Source: CAD feature listing. Evaluate the final solid. Frame: model axes, mm. Face numbers are marked on the shaded views. A direction names the side the tool comes from. Give positions to 0.01 mm unless a question says otherwise; leave off trailing zeros. Loops run counter-clockwise (first coordinate to the right, second up) from the corner with the lowest first, then second, coordinate; pieces in that order, holes last. Notation, with made-up numbers: M 50,28.25 L 63,28.25 A17 ccw 63,50.25 Z; hole C 7,29.5 d8. An arc over 180 degrees is marked long. Put each result on its own line as item: value.
from build123d import *

# Parameters (mm, degrees)
F2_SIZE  = 1
F3_R     = 0.85
F4_DEPTH = 3.001
F5_R     = 1.25
F6_DEPTH = 0.8
F7_R     = 2.25
F8_DEPTH = 2.5


with BuildPart() as f1:
    # F0 (on Front) → F1 (revolve)
    with BuildSketch(Plane.XZ):
        Polygon((0, 4), (0, 0), (3.8, 0), (3.8, 5), (3, 5), (3, 8), (1.5, 8), (1.5, 4), align=None)
    revolve(axis=Axis((1.9, 0, 0), (1, 0, 0)))

    # F2
    f2_edges = [f1.edges().sort_by_distance(p)[0] for p in [
        (0, 0, -4),
    ]]
    chamfer(f2_edges, length=F2_SIZE)

    # F3 (on face) → F4 (cut, through all)
    with BuildSketch(Plane.YZ.offset(3)):
        with Locations((6.25, 0)):
            Circle(F3_R)
        with Locations((-3.125, 5.412659)):
            Circle(F3_R)
        with Locations((-3.125, -5.412659)):
            Circle(F3_R)
    extrude(amount=-F4_DEPTH, mode=Mode.SUBTRACT)

    # F5 (on face) → F6 (cut, through all)
    with BuildSketch(Plane.YZ.offset(3.8)):
        with Locations((-5, 0)):
            Circle(F5_R)
    extrude(amount=-F6_DEPTH, mode=Mode.SUBTRACT)

    # F7 (on face) → F8 (cut)
    with BuildSketch(Plane.YZ.offset(3.8)):
        Circle(F7_R)
    extrude(amount=-F8_DEPTH, mode=Mode.SUBTRACT)


solid = f1.part
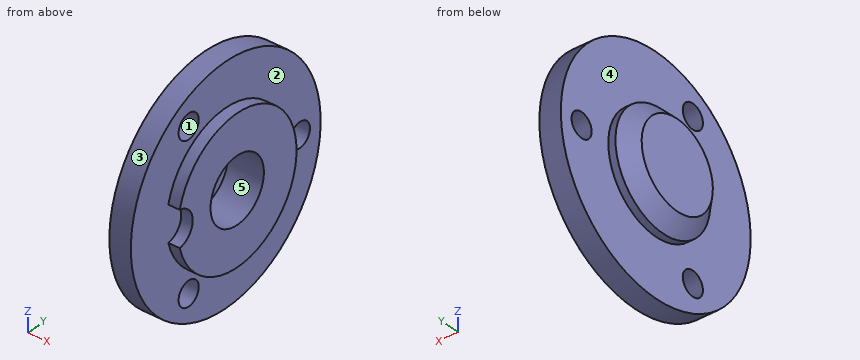
1. Access query for the marked faces 1 and 2. Directions: +Z, -Z, +X, -X, +Y, -Y. A direction counts if a zero-diameter tool reaches every point of the face in a straight line with its end or side. Return the directions, or none.
Found:
face 1: +X, -X
face 2: +X
2. Draft query along Z for the marked faces 3, 4 and 5. Return one class per face: pulls with the +Z half, pulls with the -Z half, needs draft (parallel to the pull), parting line crosses it, or undercut.
Found:
face 3: parting line crosses it
face 4: needs draft
face 5: undercut
3. Contact query for flat-ended pins moving along their axis: P1, Ø1, axis at y = -3.12, z = 5.41, coming from the -X side; P2, Ø1.3, axis at y = -1, z = 1, coming from the +X side; P3, Ø2, axis at y = -3.12, z = -5.41, coming from the -X side. Output: stop coordinate, or through.
Found:
P1: through
P2: x = 1.3
P3: x = 1.5
4. Section query D-D (y = 6.25). Output: boundary loops of the cut face in (x, z), plus the area to 3 significant figures.
Found:
outline: M 1.5,-4.99 L 3,-4.99 L 3,-0.85 L 1.5,-0.85 Z; M 1.5,0.85 L 3,0.85 L 3,4.99 L 1.5,4.99 Z
area: 12.4 mm^2
5. Section query C-C (x = 2.2). Output: boundary loops of the cut face in (y, z) (3 decimals).
Found:
outline: C 0,0 d16; hole C -3.125,-5.413 d1.7; hole C -3.125,5.413 d1.7; hole C 0,0 d4.5; hole C 6.25,0 d1.7
6. Section query B-B (y = 0). Output: boundary loops of the cut face in (x, z).
Found:
outline: M 0,-3 L 1,-4 L 1.5,-4 L 1.5,-8 L 3,-8 L 3,-5 L 3.8,-5 L 3.8,-2.25 L 1.3,-2.25 L 1.3,2.25 L 3.8,2.25 L 3.8,5 L 3,5 L 3,8 L 1.5,8 L 1.5,4 L 1,4 L 0,3 Z
7. Section query A-A (z = 0). Output: boundary loops of the cut face in (x, y).
Found:
outline: M 0,-3 L 1,-4 L 1.5,-4 L 1.5,-8 L 3,-8 L 3,-3.75 L 3.8,-3.75 L 3.8,-2.25 L 1.3,-2.25 L 1.3,2.25 L 3.8,2.25 L 3.8,5 L 3,5 L 3,5.4 L 1.5,5.4 L 1.5,4 L 1,4 L 0,3 Z; M 1.5,7.1 L 3,7.1 L 3,8 L 1.5,8 Z
8. Material intervals for line 1 (Z direction, x = 2.75, y = 0); line 2 (Z direction, x = 2.8, y = -3.75); line 3 (Y direction, x = 2.5, z = 0.5), sorted ascending. Write a range as from..to.
Found:
line 1: -8..-2.25, 2.25..8
line 2: -7.07..-5.99, -4.84..4.84, 5.99..7.07
line 3: -7.98..-2.19, 2.19..5.56, 6.94..7.98
